Read the model definition and answer for the solid it produces. Units are mm, in the model's axes. Face numbers are marked on the shaded views. A direction names the side the tool comes from. Coordinates: 2 decimals unless noted, no trailing zeros. Loops run counter-clockwise (first coordinate to the right, second up) from the corner with the lowest first, then second, coordinate; pieces in that order, holes last. Notation, with made-up numbers: M 68,24.25 L 118,24.25 A20 ccw 118,37.25 Z; hole C 11,44.5 d8. An arc over 180 degrees is marked long. Put each result on its own line as item: value.
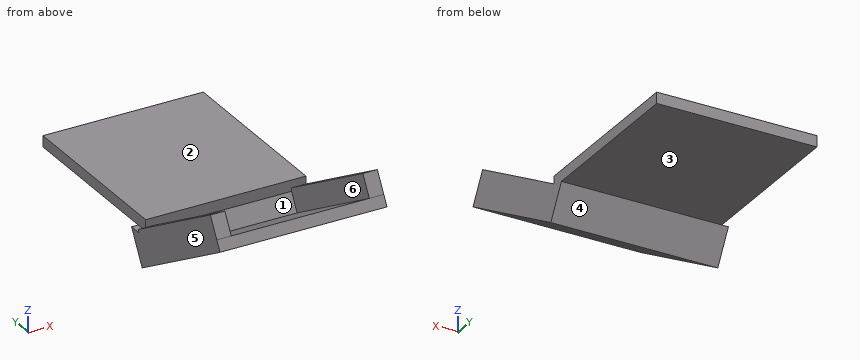
from build123d import *

# Parameters (mm, degrees)
SKIZZE1_W                       = 14.4
SKIZZE1_H                       = 16
AUFSATZ_LINEAR_AUSTRAGEN1_DEPTH = 1
AUFSATZ_LINEAR_AUSTRAGEN4_DEPTH = 15
SKIZZE9_W                       = 1.3
SKIZZE9_H                       = 13
AUFSATZ_LINEAR_AUSTRAGEN5_DEPTH = 2


with BuildPart() as part:
    # Skizze1 → Aufsatz-Linear austragen1 (new body)
    with BuildSketch(Plane.XY):
        with Locations((7.2, 8)):
            Rectangle(SKIZZE1_W, SKIZZE1_H)
    extrude(amount=AUFSATZ_LINEAR_AUSTRAGEN1_DEPTH)

    # Skizze4 → Aufsatz-Linear austragen4 (add)
    with BuildSketch(Plane(origin=(14.4, 0, 0), x_dir=(0, 0, -1), z_dir=(1, 0, 0))):
        Polygon((0, 1.154700538), (0, 0), (1.5, -0.866025404), (-5, -12.124355653), (-4.133974596, -12.624355653), (2.866025404, -0.5), align=None)
    extrude(amount=-AUFSATZ_LINEAR_AUSTRAGEN4_DEPTH)

    # Skizze9 → Aufsatz-Linear austragen5 (add)
    with BuildSketch(Plane(origin=(0, -0.866025404, -1.5), x_dir=(1, 0, 0), z_dir=(0, 0.49999999999999484, 0.8660254037844418))):
        with Locations((13.75, -6.5)):
            Rectangle(SKIZZE9_W, SKIZZE9_H)
        with Locations((0.05, -6.5)):
            Rectangle(SKIZZE9_W, SKIZZE9_H)
    extrude(amount=AUFSATZ_LINEAR_AUSTRAGEN5_DEPTH)


solid = part.part
1) Determine the mould class of the marked faces 4, 5 and 6 for opening direction Y: released by +Y, released by -Y, zero draft, split by the parting line, or undercut.
Answer list:
face 4: released by +Y
face 5: zero draft
face 6: undercut
2) Find section C-C, the plane z = 2.25. Write down the section's boundary in (x, y), plus the area to 3 significant figures.
Answer list:
outline: M -0.6,-9.36 L 14.4,-9.36 L 14.4,-3.36 L 13.1,-3.36 L 13.1,-7.36 L 0.7,-7.36 L 0.7,-3.36 L -0.6,-3.36 Z
area: 40.4 mm^2
3) Given pin 1 Ø1 at (x, y) = (10, 9.5) entering from +Z; pin 2 Ø0.5 at (x, z) = (5.5, 0.5) entering from -Y; pin 3 Ø0.8 at (y, z) = (6.5, 0.5) entering from -X; pin 4 Ø5 at (x, z) = (4, 2) entering from -Y, each flat-ended and moving along its own axis, determine where each tip first touches the part or whether it passes through.
Answer list:
pin 1: stops at z = 1
pin 2: stops at y = -6.76
pin 3: stops at x = 0
pin 4: stops at y = -12.62
4) Straight lines are drawn through the part: line 1 (Z direction, x = 0.5, y = 5); line 2 (Y direction, x = 7.5, z = 0.5); line 3 (Z direction, x = 1.75, y = -11). For each, find the intervals that lie inside material, in ascending order. Write a range as [from, to].
Answer list:
line 1: z = [0, 1]
line 2: y = [-6.33, -4.33], [0, 16]
line 3: z = [3.2, 4.35]
5) Find section B-B, the plane y = 4. Write down the section's boundary in (x, z).
Answer list:
outline: M 0,0 L 14.4,0 L 14.4,1 L 0,1 Z
6) Find section A-A, the plane x = 6. Write down the section's boundary in (y, z).
Answer list:
outline: M -12.62,4.13 L -0.5,-2.87 L 1.15,0 L 16,0 L 16,1 L 0,1 L 0,0 L -0.87,-1.5 L -12.12,5 Z
7) Find section D-D, the plane z = -2. Write down the section's boundary in (x, y), plus the area to 3 significant figures.
Answer list:
outline: M -0.6,-2 L 14.4,-2 L 14.4,0 L -0.6,0 Z
area: 30.0 mm^2
8) Which of the six approach directions +Z, -Z, +X, -X, +Y, -Y give full straight-line access (tool end or side, diameter ignored) to the marked faces 1, 2 and 3?
Answer list:
face 1: +Z
face 2: +Z, +X, -X, +Y
face 3: -Z, +X, -X, +Y
